from build123d import *

# Parameters (mm, degrees)
BOSS_EXTRUDE1_DEPTH                          = 11.5
BOSS_EXTRUDE1_TAPER                          = 2
BOSS_EXTRUDE1_OTHER_WAY_DEPTH                = 11.5
BOSS_EXTRUDE1_OTHER_WAY_TAPER                = 2
SKETCH5_R                                    = 5.125
CUT_EXTRUDE3_DEPTH                           = 76.659835157
SKETCH4_R                                    = 44
SKETCH4_R_2                                  = 41.375
CUT_EXTRUDE2_DEPTH                           = 1.75
CBORE_FOR_M5_HEX_SOCKET_HEAD_CAP_SCR_2_COUNT = 2
CBORE_FOR_M5_HEX_SOCKET_HEAD_CAP_SCR_2_PITCH = 101.5


with BuildPart() as part:
    # Sketch2 → Boss-Extrude1 (new body)
    with BuildSketch(Plane(origin=(0, 0, 0), x_dir=(1, 0, 0), z_dir=(0, 1, 0))):
        with BuildLine():
            ThreePointArc((1.131558067, 50.871129935), (0, 50.935357376), (-1.131558067, 50.871129935))
            Line((-1.131558067, 50.871129935), (-37.881558067, 46.685772559))
            ThreePointArc((-37.881558067, 46.685772559), (-43.821067812, 43.821067812), (-46.685772559, 37.881558067))
            Line((-46.685772559, 37.881558067), (-51, 0))
            Line((-51, 0), (-46.685772559, -37.881558067))
            ThreePointArc((-46.685772559, -37.881558067), (-43.821067812, -43.821067812), (-37.881558067, -46.685772559))
            Line((-37.881558067, -46.685772559), (-1.131558067, -50.871129935))
            ThreePointArc((-1.131558067, -50.871129935), (0, -50.935357376), (1.131558067, -50.871129935))
            Line((1.131558067, -50.871129935), (37.881558067, -46.685772559))
            ThreePointArc((37.881558067, -46.685772559), (43.821067812, -43.821067812), (46.685772559, -37.881558067))
            Line((46.685772559, -37.881558067), (51, 0))
            Line((51, 0), (46.685772559, 37.881558067))
            ThreePointArc((46.685772559, 37.881558067), (43.821067812, 43.821067812), (37.881558067, 46.685772559))
            Line((37.881558067, 46.685772559), (1.131558067, 50.871129935))
        make_face()
    extrude(amount=BOSS_EXTRUDE1_DEPTH, taper=BOSS_EXTRUDE1_TAPER)

    # Sketch2 → Boss-Extrude1 other way (add)
    with BuildSketch(Plane(origin=(0, 0, 0), x_dir=(1, 0, 0), z_dir=(0, 1, 0))):
        with BuildLine():
            ThreePointArc((1.131558067, 50.871129935), (0, 50.935357376), (-1.131558067, 50.871129935))
            Line((-1.131558067, 50.871129935), (-37.881558067, 46.685772559))
            ThreePointArc((-37.881558067, 46.685772559), (-43.821067812, 43.821067812), (-46.685772559, 37.881558067))
            Line((-46.685772559, 37.881558067), (-51, 0))
            Line((-51, 0), (-46.685772559, -37.881558067))
            ThreePointArc((-46.685772559, -37.881558067), (-43.821067812, -43.821067812), (-37.881558067, -46.685772559))
            Line((-37.881558067, -46.685772559), (-1.131558067, -50.871129935))
            ThreePointArc((-1.131558067, -50.871129935), (0, -50.935357376), (1.131558067, -50.871129935))
            Line((1.131558067, -50.871129935), (37.881558067, -46.685772559))
            ThreePointArc((37.881558067, -46.685772559), (43.821067812, -43.821067812), (46.685772559, -37.881558067))
            Line((46.685772559, -37.881558067), (51, 0))
            Line((51, 0), (46.685772559, 37.881558067))
            ThreePointArc((46.685772559, 37.881558067), (43.821067812, 43.821067812), (37.881558067, 46.685772559))
            Line((37.881558067, 46.685772559), (1.131558067, 50.871129935))
        make_face()
    extrude(amount=-BOSS_EXTRUDE1_OTHER_WAY_DEPTH, taper=BOSS_EXTRUDE1_OTHER_WAY_TAPER)

    # Sketch5 → Cut-Extrude3 (cut, through all)
    with BuildSketch(Plane.XZ.offset(11.5)):
        with Locations(Location((-36.75, 36.75, 0), (0, 0, 270))):
            Circle(SKETCH5_R)
        with Locations(Location((36.75, 36.75, 0), (0, 0, 270))):
            Circle(SKETCH5_R)
        with Locations(Location((-36.75, -36.75, 0), (0, 0, 270))):
            Circle(SKETCH5_R)
        with Locations(Location((36.75, -36.75, 0), (0, 0, 270))):
            Circle(SKETCH5_R)
    extrude(amount=-CUT_EXTRUDE3_DEPTH, mode=Mode.SUBTRACT)

    # Sketch4 → Cut-Extrude2 (cut)
    with BuildSketch(Plane.XZ.offset(11.5)):
        with Locations(Location((0, 0, 0), (0, 0, 270))):
            Circle(SKETCH4_R)
        with Locations(Location((0, 0, 0), (0, 0, 270))):
            Circle(SKETCH4_R_2, mode=Mode.SUBTRACT)
    extrude(amount=-CUT_EXTRUDE2_DEPTH, mode=Mode.SUBTRACT)

    # Sketch6 → Cut-Revolve1 (revolve, cut)
    with BuildSketch(Plane(origin=(0, 0, 0), x_dir=(0, 0, -1), z_dir=(1, 0, 0)), mode=Mode.PRIVATE) as cut_revolve1_sk:
        with BuildLine():
            Line((37.45, 10.5), (37.45, 4.9))
            ThreePointArc((37.45, 4.9), (37.567157288, 4.617157288), (37.85, 4.5))
            Line((37.85, 4.5), (75, 4.5))
            Line((75, 4.5), (75, 13.5))
            Line((75, 13.5), (0, 13.5))
            Line((0, 13.5), (0, -11.5))
            Line((0, -11.5), (17, -11.5))
            Line((17, -11.5), (15, -9.5))
            Line((15, -9.5), (15, 8))
            ThreePointArc((15, 8), (15.146446609, 8.353553391), (15.5, 8.5))
            Line((15.5, 8.5), (19.7, 8.5))
            ThreePointArc((19.7, 8.5), (19.982842712, 8.617157288), (20.1, 8.9))
            Line((20.1, 8.9), (20.1, 11.3))
            ThreePointArc((20.1, 11.3), (20.158578644, 11.441421356), (20.3, 11.5))
            Line((20.3, 11.5), (36.45, 11.5))
            Line((36.45, 11.5), (37.45, 10.5))
        make_face()
    revolve(cut_revolve1_sk.sketch.rotate(Axis((0, 29.196100586, 0), (0, -1, 0)), 180), axis=Axis((0, 29.196100586, 0), (0, -1, 0)), mode=Mode.SUBTRACT)

    # Sketch9 → Cut-Revolve2 (revolve, cut)
    with BuildSketch(Plane.XY, mode=Mode.PRIVATE) as cut_revolve2_sk:
        Polygon((-37.34396054, -12.765501422), (-23.84396054, 10.234498578), (-22.346696913, 12.785392166), (-24.502736372, 14.050893588), (-43.54960455, -18.399326271), (-41.393565091, -19.664827692), align=None)
    revolve(cut_revolve2_sk.sketch.rotate(Axis((-43.54960455, -18.399326271, 0), (0.5062005687642237, 0.8624157838205285, 0)), 230.866713555), axis=Axis((-43.54960455, -18.399326271, 0), (0.5062005687642237, 0.8624157838205285, 0)), mode=Mode.SUBTRACT)

    # Sketch12 → CBORE for M5 Hex Socket Head Cap Screw1 (revolve, cut)
    with BuildSketch(Plane(origin=(26.89340266, 4.5, -43.03844088), x_dir=(0, 0, 1), z_dir=(1, 0, 0))):
        Polygon((0, 0), (0, 16), (2.775, 16), (2.75, 15.975), (2.75, 6.325), (2.775, 6.3), (4.5, 6.3), (4.5, 0), align=None)
    cbore_for_m5_hex_socket_head_cap_screw1 = revolve(axis=Axis((26.89340266, 10.85, -43.03844088), (0, -1, 0)), mode=Mode.SUBTRACT)

    # CBORE for M5 Hex Socket Head Cap Scr 2: CBORE for M5 Hex Socket Head Cap Screw1 ×2
    with Locations(*[Vector(-0.5299192642331998, 0, 0.8480480961564293) * (i * CBORE_FOR_M5_HEX_SOCKET_HEAD_CAP_SCR_2_PITCH) for i in range(1, CBORE_FOR_M5_HEX_SOCKET_HEAD_CAP_SCR_2_COUNT)]):
        add(cbore_for_m5_hex_socket_head_cap_screw1, mode=Mode.SUBTRACT)


solid = part.part
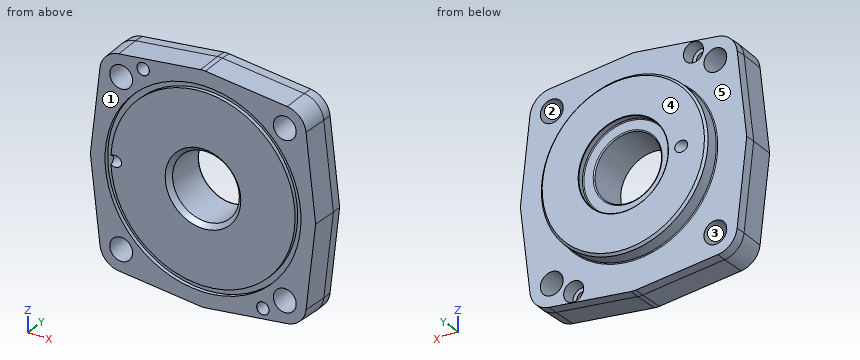
Read the model definition and answer for the solid it produces. Units are mm, in the model's axes. Face numbers are marked on the shaded views. A direction names the side the tool comes from. Round coordinates to 2 decimals unless told otherwise and drop trailing zeros.
1. Given pin 1 Ø16.5 at (x, z) = (36.75, -36.75) entering from +Y; pin 2 Ø2 at (y, z) = (6.5, 17) entering from -X; pin 3 Ø12 at (x, y) = (-18.5, 6.5) entering from +Z; pin 4 Ø24 at (x, z) = (0, 0) entering from +Y, each flat-ended and moving along its own axis, determine where each tip first touches the part or whether it passes through.
2. Straight lines are drawn through the part: L1, parallel to Z at x = -39, y = -8.25; L2, parallel to X at y = 0.25, z = 2; L3, parallel to X at y = 1, z = -33. For each, find the intervals that lie inside material, in ascending order.
3. Which of the six approach directions +Z, -Z, +X, -X, +Y, -Y give full straight-line access (tool end or side, diameter ignored) to the marked faces 4 and 5?
4. Determine the mould class of the marked faces 1, 2 and 3 for opening direction X: pulls with the +X half, pulls with the -X half, needs draft (parallel to the pull), parting line crosses it, or undercut.
5. The part is cut by section A-A, the plane y = 1.25. State how many separate pieces and enclosed holes the cut face has, then the cut area to 3 significant figures.
Values:
1. pin 1: stops at y = 4.5
1. pin 2: stops at x = -33.86
1. pin 3: stops at z = 49.38
1. pin 4: passes through
2. L1: z = -46.2 to -41.35, -32.15 to -2.19, 2.19 to 32.15, 41.35 to 46.2
2. L2: x = -50.76 to -34.34, -30.86 to -14.87, 14.87 to 50.76
2. L3: x = -47.21 to -40.24, -33.26 to 33.26, 40.24 to 47.21
3. face 4: +Z, -Z, +X, -X, +Y
3. face 5: +Y
4. face 1: needs draft
4. face 2: undercut
4. face 3: undercut
5. separate pieces: 1
5. enclosed holes: 8
5. area: 8,090 mm2
